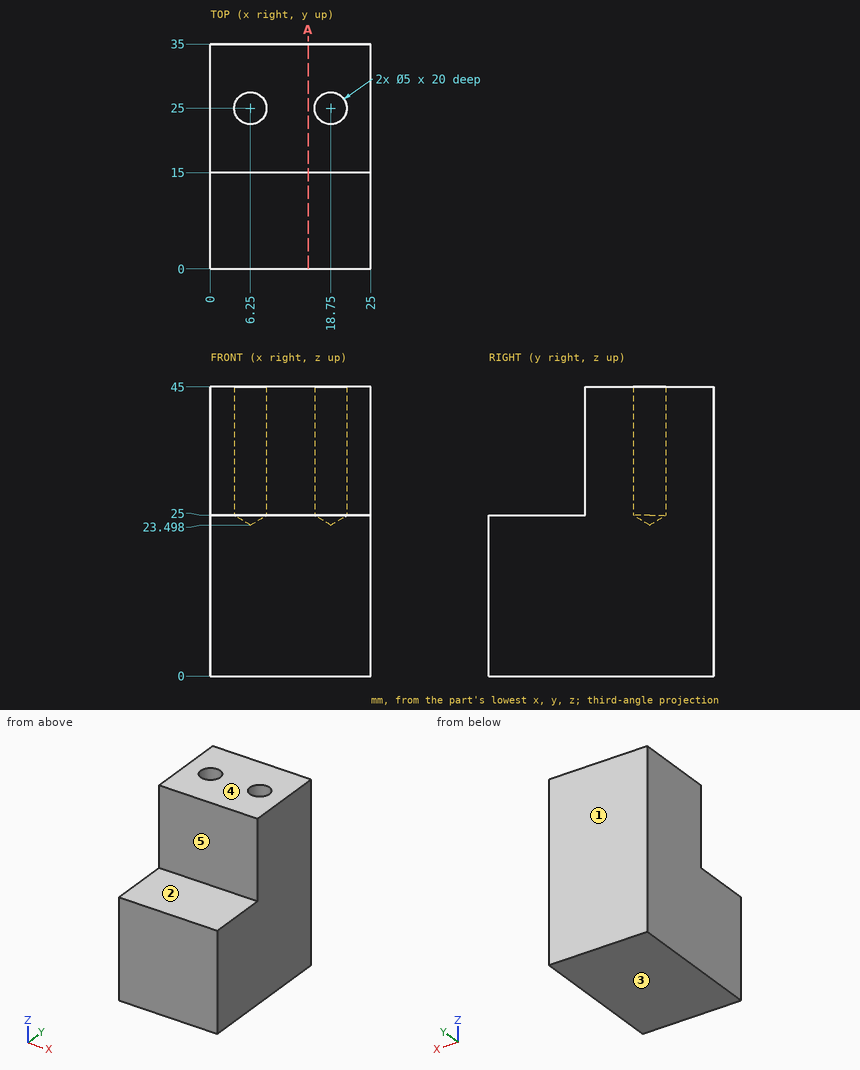
Check sheet for the drawn part. Datum: minimum x, y, z corner. Units: mm. A direction names the side the tool comes from. Round coordinates to 2 decimals unless told otherwise and drop trailing zeros. Order: outer loops, then holes, each group sorted by start corner. A loop starts at its lowest first (then second) coordinate and runs counter-clockwise, first axis right, second up. Notation, with made-up numbers: (53, 83) -> (96, 83) arc R21 cw to (96, 89) -> close; hole circle Ø6 at (42, -19). An arc over 180 degrees is marked (long way). Return JSON: item names as keys, results as strings. Group by question number.
Q1. Tool access check on the marked faces 4 and 5. Record the directions out of +Z, -Z, +X, -X, +Y, -Y that give a thin tool (end or side, any length) a straight path to the whole face; none if there is none.
Q2. Section check A-A, the plane x = 15.25. Record the boundary of the cut face in (y, z).
Q3. Release check for a two-part mould opening along Z. For the marked faces 1, 2 and 3 record: released by +Z, released by -Z, zero draft, split by the parting line, or undercut.
Q4. Material ranges on probe 1 along X at (y, z) = (25, 32); probe 2 along Y at (x, z) = (6.25, 34.5); probe 3 along Y at (x, z) = (9.75, 42.5), recorded low to high. Write a range as from..to.
Q5. Gauge pin test, flat ends, axial feed: pin 1 (8 mm diameter, centred on y = 16.5, z = 8, fed in from -X); pin 2 (4.5 mm diameter, centred on x = 6.25, y = 25, fed in from +Z); pin 3 (3 mm diameter, centred on x = 21, y = 9, fed in from +Z). Record the tip position at first contact, or that the pin passes through.
Numbers:
{
 "1": {"face 4": "+Z, +X, -X, +Y, -Y", "face 5": "+Z, +X, -X, -Y"},
 "2": {"outline": "(0, 0) -> (35, 0) -> (35, 45) -> (15, 45) -> (15, 25) -> (0, 25) -> close"},
 "3": {"face 1": "zero draft", "face 2": "released by +Z", "face 3": "released by -Z"},
 "4": {"probe 1": "0..3.75, 8.75..16.25, 21.25..25", "probe 2": "15..22.5, 27.5..35", "probe 3": "15..35"},
 "5": {"pin 1": "x = 0", "pin 2": "z = 24.85", "pin 3": "z = 25"}
}
